```python
from build123d import *

# Parameters (mm, degrees)
BOSS_EXTRUDE1_DEPTH     = 3
SKETCH3_R               = 1.6
CUT_EXTRUDE1_DEPTH      = 3
CHAMFER1_SIZE           = 1.8
SKETCH5_W               = 26
SKETCH5_H               = 26
SKETCH5_W_2             = 8.5
SKETCH5_H_2             = 8.5
CUT_EXTRUDE2_DEPTH      = 3
CHAMFER2_SIZE           = 1.5
SKETCH7_W               = 3.5
SKETCH7_H               = 11.5
BOSS_EXTRUDE3_DEPTH     = 6.2
CUT_EXTRUDE3_DEPTH      = 125.687357779
CUT_EXTRUDE3_DEPTH_BACK = 3
CHAMFER3_SIZE           = 1
SKETCH9_W               = 25
SKETCH9_H               = 4
SKETCH9_W_2             = 4
SKETCH9_H_2             = 5
BOSS_EXTRUDE4_DEPTH     = 1.9
BOSS_EXTRUDE5_DEPTH     = 5.5
SKETCH11_W              = 4
SKETCH11_H              = 17.5
BOSS_EXTRUDE6_DEPTH     = 3.5
BOSS_EXTRUDE7_DEPTH     = 4.5
SKETCH13_W              = 3.4
SKETCH13_H              = 16.58647312
BOSS_EXTRUDE8_DEPTH     = 2
SKETCH14_W              = 10
SKETCH14_H              = 3
CUT_EXTRUDE4_DEPTH      = 3
CHAMFER4_SIZE           = 1


with BuildPart() as part:
    # Sketch1 → Boss-Extrude1 (new body)
    with BuildSketch(Plane.XY):
        Polygon((0.01715505, 91.462274694), (84.51715505, 91.462274694), (84.51715505, 83.862274694), (74.51715505, 73.862274694), (74.51715505, 32.562274694), (84.51715505, 22.562274694), (84.51715505, -0.037725306), (71.91715505, -0.037725306), (61.91715505, 9.962274694), (22.61715505, 9.962274694), (12.61715505, -0.037725306), (0.01715505, -0.037725306), align=None)
    extrude(amount=BOSS_EXTRUDE1_DEPTH)

    # Sketch3 → Cut-Extrude1 (cut)
    with BuildSketch(Plane.XY.offset(3)):
        with Locations((5.26715505, 86.212274694)):
            Circle(SKETCH3_R)
        with Locations((79.26715505, 86.212274694)):
            Circle(SKETCH3_R)
        with Locations((5.26715505, 5.212274694)):
            Circle(SKETCH3_R)
        with Locations((79.26715505, 5.212274694)):
            Circle(SKETCH3_R)
    extrude(amount=-CUT_EXTRUDE1_DEPTH, mode=Mode.SUBTRACT)

    # Chamfer1
    chamfer1_edges = [part.edges().sort_by_distance(p)[0] for p in [
        (77.66715505, 86.212274694, 3),
        (3.66715505, 5.212274694, 3),
        (77.66715505, 5.212274694, 3),
        (3.66715505, 86.212274694, 3),
    ]]
    chamfer(chamfer1_edges, length=CHAMFER1_SIZE)

    # Sketch5 → Cut-Extrude2 (cut)
    with BuildSketch(Plane.XY.offset(3)):
        with Locations((35.51715505, 59.962274694)):
            Rectangle(SKETCH5_W, SKETCH5_H)
        with Locations((61.41715505, 70.562274694)):
            Rectangle(SKETCH5_W_2, SKETCH5_H_2)
    extrude(amount=-CUT_EXTRUDE2_DEPTH, mode=Mode.SUBTRACT)

    # Chamfer2
    chamfer2_edges = [part.edges().sort_by_distance(p)[0] for p in [
        (57.16715505, 70.562274694, 3),
        (61.41715505, 66.312274694, 3),
        (65.66715505, 70.562274694, 3),
        (61.41715505, 74.812274694, 3),
        (22.51715505, 59.962274694, 3),
        (35.51715505, 46.962274694, 3),
        (48.51715505, 59.962274694, 3),
        (35.51715505, 72.962274694, 3),
    ]]
    chamfer(chamfer2_edges, length=CHAMFER2_SIZE)

    # Sketch7 → Boss-Extrude3 (add)
    with BuildSketch(Plane.XY.offset(3)):
        with Locations((74.51715505, 52.762274694)):
            Rectangle(SKETCH7_W, SKETCH7_H)
    extrude(amount=-BOSS_EXTRUDE3_DEPTH)

    # Sketch8 → Cut-Extrude3 (cut, two sides: drawn at the far end of the back side and taken through both)
    with BuildSketch(Plane(origin=(0, 0, -3.2), x_dir=(-1, 0, 0), z_dir=(0, 0, -1)).offset(-CUT_EXTRUDE3_DEPTH_BACK)):
        with BuildLine():
            Line((-76.26715505, 58.512274694), (-76.26715505, 47.012274694))
            ThreePointArc((-76.26715505, 47.012274694), (-75.034557132, 52.762274694), (-76.26715505, 58.512274694))
        make_face()
    extrude(amount=CUT_EXTRUDE3_DEPTH + CUT_EXTRUDE3_DEPTH_BACK, mode=Mode.SUBTRACT)

    # Chamfer3
    # the kernel refuses this chamfer: 1 mm, written as the material it takes off along each edge
    with BuildSketch(Plane(origin=(76.26715505, 61.083957682, -0.2), x_dir=(0.02749587661058217, 0, 0.9996219169112968), z_dir=(0, -1, 0))) as chamfer3_piece_1_section:
        Polygon((CHAMFER3_SIZE * 0.999621916911, CHAMFER3_SIZE * 0.0274958766106), (-CHAMFER3_SIZE * 0.0274958766106, CHAMFER3_SIZE * 0.999621916911), (0, 0), align=None)
    chamfer3_piece_1 = extrude(amount=16.643365976, mode=Mode.PRIVATE)
    chamfer3_piece_1 = chamfer3_piece_1 & Plane(origin=(89.06256948, 52.762274694, 0.149616296), x_dir=(-0.9121331028647569, -0.4098941359159838, 0), z_dir=(0, 0, 1)) * Cylinder(14.028012348, 38, mode=Mode.PRIVATE)
    add(chamfer3_piece_1, mode=Mode.SUBTRACT)

    # Sketch9 → Boss-Extrude4 (add)
    with BuildSketch(Plane(origin=(0, 0, 0), x_dir=(-1, 0, 0), z_dir=(0, 0, -1))):
        with Locations((-35.51715505, 37.962274694)):
            Rectangle(SKETCH9_W, SKETCH9_H)
        with Locations((-48.51715505, 77.462274694)):
            Rectangle(SKETCH9_W_2, SKETCH9_H_2)
        with Locations((-22.51715505, 77.462274694)):
            Rectangle(SKETCH9_W_2, SKETCH9_H_2)
    extrude(amount=BOSS_EXTRUDE4_DEPTH)

    # Sketch10 → Boss-Extrude5 (add)
    with BuildSketch(Plane(origin=(0, 0, 0), x_dir=(-1, 0, 0), z_dir=(0, 0, -1))):
        Polygon((-21.41715505, 80.962274694), (-72.91715505, 80.962274694), (-72.91715505, 60.962274694), (-69.51715505, 60.962274694), (-69.51715505, 77.962274694), (-21.41715505, 77.962274694), align=None)
        Polygon((-72.91715505, 44.424333564), (-69.51715505, 44.424333564), (-69.51715505, 40.962274694), (-52.91715505, 40.962274694), (-52.91715505, 37.962274694), (-72.91715505, 37.962274694), align=None)
    extrude(amount=BOSS_EXTRUDE5_DEPTH)

    # Sketch11 → Boss-Extrude6 (add)
    with BuildSketch(Plane(origin=(0, 0, 0), x_dir=(-1, 0, 0), z_dir=(0, 0, -1))):
        with Locations((-26.01715505, 27.712274694)):
            Rectangle(SKETCH11_W, SKETCH11_H)
    extrude(amount=BOSS_EXTRUDE6_DEPTH)

    # Sketch12 → Boss-Extrude7 (add)
    with BuildSketch(Plane(origin=(0, 0, 0), x_dir=(-1, 0, 0), z_dir=(0, 0, -1))):
        Polygon((-19.71715505, 79.962274694), (-1.71715505, 79.962274694), (-1.71715505, 72.462274694), (-1.71715505, 19.462274694), (-1.71715505, 11.462274694), (-19.71715505, 11.462274694), (-19.71715505, 19.462274694), (-3.71715505, 19.462274694), (-3.71715505, 71.962274694), (-19.71715505, 71.962274694), align=None)
    extrude(amount=BOSS_EXTRUDE7_DEPTH)

    # Sketch13 → Boss-Extrude8 (add)
    with BuildSketch(Plane(origin=(0, 0, 0), x_dir=(-1, 0, 0), z_dir=(0, 0, -1))):
        Polygon((-18.51715505, 77.962274694), (-21.91715505, 77.962274694), (-21.91715505, 86.862274694), (-69.91715505, 86.862274694), (-69.91715505, 80.962274694), (-72.91715505, 80.962274694), (-72.91715505, 89.862274694), (-18.51715505, 89.862274694), align=None)
        Polygon((-72.91715505, 37.962274694), (-69.91715505, 37.962274694), (-69.91715505, 14.562274694), (-1.61715505, 14.562274694), (-1.61715505, 11.562274694), (-72.91715505, 11.562274694), align=None)
        with Locations((-71.21715505, 52.669038134)):
            Rectangle(SKETCH13_W, SKETCH13_H)
    extrude(amount=BOSS_EXTRUDE8_DEPTH)

    # Sketch14 → Cut-Extrude4 (cut)
    with BuildSketch(Plane(origin=(0, 0, 0), x_dir=(-1, 0, 0), z_dir=(0, 0, -1))):
        with Locations((-37.91715505, 20.062274694)):
            Rectangle(SKETCH14_W, SKETCH14_H)
        with Locations((-59.91715505, 20.062274694)):
            Rectangle(SKETCH14_W, SKETCH14_H)
        with Locations((-37.91715505, 28.062274694)):
            Rectangle(SKETCH14_W, SKETCH14_H)
        with Locations((-59.91715505, 28.062274694)):
            Rectangle(SKETCH14_W, SKETCH14_H)
    extrude(amount=-CUT_EXTRUDE4_DEPTH, mode=Mode.SUBTRACT)

    # Chamfer4
    chamfer4_edges = [part.edges().sort_by_distance(p)[0] for p in [
        (76.26715505, 52.762274694, 3),
    ]]
    chamfer(chamfer4_edges, length=CHAMFER4_SIZE)


solid = part.part
```
The listing builds one solid part. Answer for the finished solid, in the listing's coordinates (mm). A direction names the side the tool comes from. Give positions to 0.01 mm unless a question says otherwise; leave off trailing zeros. Order: outer loops, then holes, each group sorted by start corner. A loop starts at its lowest first (then second) coordinate and runs counter-clockwise, first axis right, second up. Notation, with made-up numbers: (9.5, -21.75) -> (55.5, -21.75) arc R25 cw to (55.5, -5.75) -> close; hole circle Ø1 at (68.25, -7). An arc over 180 degrees is marked (long way). Answer as CSV lines item,"result". Start each with the question number.
Q1. Find the intervals of material crossed by L1, parallel to Y at x = 56.5, z = 0.25; L2, parallel to Y at x = 29, z = -0.5; L3, parallel to X at y = 75.5, z = -1, in increasing order.
Q2. A cutting plane is placed at A-A (x = 30). Determine the outline of the cut face in (y, z).
Q3. Given pin 1 (1 mm diameter, centred on x = 35, z = 1.5, fed in from -Y); pin 2 (3.5 mm diameter, centred on y = 77.5, z = -3, fed in from +X); pin 3 (2 mm diameter, centred on y = 61.5, z = -1.5, fed in from -X), each flat-ended and moving along its own axis, determine where each tip first touches the part or whether it passes through.
Q4. Which of the six approach directions +Z, -Z, +X, -X, +Y, -Y give full straight-line access (tool end or side, diameter ignored) to faces 1 (the flat face through (1.717, 45, -2)), 2 (the flat face through (69.917, 84, -1)), 3 (the flat face through (74.517, 40, 1)), 4 (the flat face through (38, 21.562, 1)), 5 (the flat face through (46, 11.562, -1))?
Q5. A cutting plane is placed at B-B (y = 52). Determine the outline of the cut face in (x, z).
Q6. Determine the mould class of faces 6 (the flat face through (84.517, 11, 1)), 7 (the flat face through (6, -0.038, 1)), 8 (the cylindrical face through (78.92, 84.65, 0.61)) for opening direction Y: pulls with the +Y half, pulls with the -Y half, needs draft (parallel to the pull), parting line crosses it, or undercut.
Results found:
1,L1,"9.96 to 18.56, 21.56 to 26.56, 29.56 to 91.46"
1,L2,"11.56 to 14.56, 35.96 to 39.96, 77.96 to 80.96, 86.86 to 89.86"
1,L3,"1.72 to 19.72, 20.52 to 24.52, 46.52 to 50.52, 69.52 to 72.92"
2,outline,"(9.96, 0) -> (11.56, 0) -> (11.56, -2) -> (14.56, -2) -> (14.56, 0) -> (35.96, 0) -> (35.96, -1.9) -> (39.96, -1.9) -> (39.96, 0) -> (46.96, 0) -> (46.96, 1.5) -> (45.46, 3) -> (9.96, 3) -> close; (72.96, 0) -> (77.96, 0) -> (77.96, -5.5) -> (80.96, -5.5) -> (80.96, 0) -> (86.86, 0) -> (86.86, -2) -> (89.86, -2) -> (89.86, 0) -> (91.46, 0) -> (91.46, 3) -> (74.46, 3) -> (72.96, 1.5) -> close"
3,pin 1,"y = 9.96"
3,pin 2,"x = 72.92"
3,pin 3,"x = 1.72"
4,face 1,"-Z, -X, +Y"
4,face 2,"-Z"
4,face 3,"+Z, -Z, +X"
4,face 4,"+Z, -Z"
4,face 5,"-Z, +X, -Y"
5,outline,"(0.02, 0) -> (1.72, 0) -> (1.72, -4.5) -> (3.72, -4.5) -> (3.72, 0) -> (22.52, 0) -> (22.52, 1.5) -> (21.02, 3) -> (0.02, 3) -> close; (48.52, 0) -> (69.52, 0) -> (69.52, -2) -> (72.77, -2) -> (72.77, -3.2) -> (75.06, -3.2) -> (75.06, -0.2) -> (75.27, -0.2) -> (76.27, 0.8) -> (76.27, 2) -> (75.27, 3) -> (50.02, 3) -> (48.52, 1.5) -> close"
6,face 6,"needs draft"
6,face 7,"pulls with the -Y half"
6,face 8,"undercut"
